The listing builds one solid part. Answer for the finished solid, in the listing's coordinates (mm). Face numbers are marked on the shaded views. Round coordinates to 2 decimals unless told otherwise and drop trailing zeros. Write each loop counter-clockwise with the first axis right and the second up, starting at its lowest first coordinate (ties: lowest second). Pieces come first, ordered by that corner, then holes.
Item 1: Find the intervals of material crossed by probe 1 along X at (y, z) = (1.75, -10.5); probe 2 along Z at (x, y) = (13.5, 2.8); probe 3 along X at (y, z) = (1.25, 13), in increasing order.
Item 2: Find section B-B on x = 15. Give the vertices of the cut face in (y, z).
Item 3: For a pull along Z with two mould halves and no side action, classify the marked faces 1 and 2 as +Z half, -Z half, draft (parallel to the pull), parting line (faces both ways), or undercut.
Item 4: Each of these flat-tipped pins is pushed along its axis until it touches: pin 1 (5 mm diameter, centred on x = 3, z = -1, fed in from -Y); pin 2 (4.5 mm diameter, centred on x = 15, z = -10.5, fed in from +Y). Where does it stop, or does it pass through?
Item 5: Find section C-C on y = 1.75. Give the vertices of the cut face in (x, z), then the cut area to 3 significant figures.
Item 6: Find section D-D on z = 3. Give the vertices of the cut face in (x, y) (3 decimals), then the cut area to 3 significant figures.
Item 7: Find section A-A on z = -10.5. Give the vertices of the cut face in (x, y), then the cut area to 3 significant figures.
```python
from build123d import *

# Parameters (mm, degrees)
SKETCH1_W           = 40
SKETCH1_H           = 31
BOSS_EXTRUDE1_DEPTH = 3
SKETCH2_R           = 2.75
CUT_EXTRUDE1_DEPTH  = 3
SKETCH3_R           = 8.725
CUT_EXTRUDE2_DEPTH  = 0.5
SKETCH4_R           = 4
CUT_EXTRUDE3_DEPTH  = 2.5


with BuildPart() as part:
    # Sketch1 → Boss-Extrude1 (new body)
    with BuildSketch(Plane(origin=(0, 0, 0), x_dir=(1, 0, 0), z_dir=(0, 1, 0))):
        Rectangle(SKETCH1_W, SKETCH1_H)
    extrude(amount=BOSS_EXTRUDE1_DEPTH)

    # Sketch2 → Cut-Extrude1 (cut)
    with BuildSketch(Plane(origin=(0, 3, 0), x_dir=(1, 0, 0), z_dir=(0, 1, 0))):
        with Locations(Location((-15, 10.5, 0), (0, 0, 270))):
            Circle(SKETCH2_R)
        with Locations(Location((15, 10.5, 0), (0, 0, 270))):
            Circle(SKETCH2_R)
        with Locations(Location((15, -10.5, 0), (0, 0, 270))):
            Circle(SKETCH2_R)
        with Locations(Location((-15, -10.5, 0), (0, 0, 270))):
            Circle(SKETCH2_R)
    extrude(amount=-CUT_EXTRUDE1_DEPTH, mode=Mode.SUBTRACT)

    # Sketch3 → Cut-Extrude2 (cut)
    with BuildSketch(Plane.XZ):
        with Locations(Location((0, 3, 0), (0, 0, 270))):
            Circle(SKETCH3_R)
    extrude(amount=-CUT_EXTRUDE2_DEPTH, mode=Mode.SUBTRACT)

    # Sketch4 → Cut-Extrude3 (cut)
    with BuildSketch(Plane(origin=(0, 3, 0), x_dir=(1, 0, 0), z_dir=(0, 1, 0))):
        with Locations(Location((0, -3, 0), (0, 0, 270))):
            Circle(SKETCH4_R)
    extrude(amount=-CUT_EXTRUDE3_DEPTH, mode=Mode.SUBTRACT)


solid = part.part
```
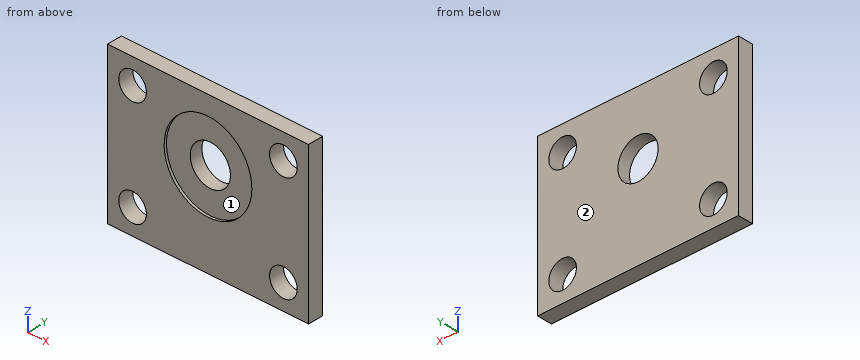
Check values:
1. probe 1: x = -20 to -17.75, -12.25 to 12.25, 17.75 to 20
1. probe 2: z = -15.5 to -12.8, -8.2 to 8.2, 12.8 to 15.5
1. probe 3: x = -20 to -16.15, -13.85 to 13.85, 16.15 to 20
2. outline: (0, -15.5) - (3, -15.5) - (3, -13.25) - (0, -13.25) - close; (0, -7.75) - (3, -7.75) - (3, 7.75) - (0, 7.75) - close; (0, 13.25) - (3, 13.25) - (3, 15.5) - (0, 15.5) - close
3. face 1: undercut
3. face 2: draft
4. pin 1: stops at y = 0.5
4. pin 2: passes through
5. outline: (-20, -15.5) - (20, -15.5) - (20, 15.5) - (-20, 15.5) - close; hole circle Ø5.5 at (-15, -10.5); hole circle Ø5.5 at (-15, 10.5); hole circle Ø8 at (0, 3); hole circle Ø5.5 at (15, -10.5); hole circle Ø5.5 at (15, 10.5)
5. area: 1,090 mm2
6. outline: (-20, 0) - (-8.725, 0) - (-8.725, 0.5) - (-4, 0.5) - (-4, 3) - (-20, 3) - close; (4, 0.5) - (8.725, 0.5) - (8.725, 0) - (20, 0) - (20, 3) - (4, 3) - close
6. area: 91.3 mm2
7. outline: (-20, 0) - (-17.75, 0) - (-17.75, 3) - (-20, 3) - close; (-12.25, 0) - (12.25, 0) - (12.25, 3) - (-12.25, 3) - close; (17.75, 0) - (20, 0) - (20, 3) - (17.75, 3) - close
7. area: 87.0 mm2
